Check sheet for the modelled part. Datum: model origin and axes. Units: mm. Give positions to 0.01 mm unless a question says otherwise; leave off trailing zeros. Order: outer loops, then holes, each group sorted by start corner. A loop starts at its lowest first (then second) coordinate and runs counter-clockwise, first axis right, second up. Notation, with made-up numbers: (-17.5, 58) - (11.5, 58) arc R19 cw to (11.5, 79) - close; hole circle Ø1 at (8.25, -25.75). An arc over 180 degrees is marked (long way). Answer in a Markdown table with one row per item.
Autodesk Inventor part; units mm, degrees
ref_plane "YZ Plane" through (0, 0, 0) normal (1, 0, 0) x (0, 1, 0)
ref_plane "XZ Plane" through (0, 0, 0) normal (0, 1, 0) x (-1, 0, 0)
ref_plane "XY Plane" through (0, 0, 0) normal (0, 0, 1) x (1, 0, 0)
sketch "Sketch1" plane through (0, 0, 0) normal (0, 1, 0) x (-1, 0, 0)
  line L0 (-40, 50) -> (40, 50)
  line L1 (40, 50) -> (40, -50)
  line L2 (40, -50) -> (-40, -50)
  line L3 (-40, -50) -> (-40, 50)
  line L4 (-40, 50) -> (40, -50) construction
  line L5 (40, 50) -> (-40, -50) construction
  circle A0 centre (34.29, 45.72) radius 2
  line L6 (-34.29, 45.72) -> (34.29, 45.72) construction
  line L7 (34.29, 45.72) -> (34.29, -45.72) construction
  line L8 (34.29, -45.72) -> (-34.29, -45.72) construction
  line L9 (-34.29, -45.72) -> (-34.29, 45.72) construction
  line L10 (-34.29, 45.72) -> (34.29, -45.72) construction
  line L11 (34.29, 45.72) -> (-34.29, -45.72) construction
  circle A1 centre (34.29, -45.72) radius 2
  circle A2 centre (-34.29, -45.72) radius 2
  circle A3 centre (-34.29, 45.72) radius 2
  point P0 (0, 0)
  dimension "d0" = 100
  dimension "d1" = 80
  dimension "d2" = 4
  dimension "d15" = 91.44
  dimension "d16" = 68.58
  dimension "d17" = 4
  dimension "d18" = 4
  dimension "d19" = 4
extrude "Extrusion1" add sketch "Sketch1" along normal blind 2
properties part number "PCB" material "ABS Plastic"
(1) Cross-section at A-A, the plane x = -34.29. Record the cut outline in (y, z).
Geometry says:
| item | result |
|---|---|
| outline | (0, -50) - (2, -50) - (2, -47.72) - (0, -47.72) - close; (0, -43.72) - (2, -43.72) - (2, 43.72) - (0, 43.72) - close; (0, 47.72) - (2, 47.72) - (2, 50) - (0, 50) - close |
(2) Mould release check, pull along Z, two halves, no side actions. Record for faces 1 (the flat face through (1, 1, 50)), 2 (the flat face through (40, 1, -1)), 3 (the cylindrical face through (-34.03, 0.986, 43.737)): pulls with the +Z half, pulls with the -Z half, needs draft (parallel to the pull), parting line crosses it, or undercut.
Geometry says:
| item | result |
|---|---|
| face 1 | pulls with the +Z half |
| face 2 | needs draft |
| face 3 | undercut |
(3) Thickness scan on L1, parallel to Z at x = -34.29, y = 0.65; L2, parallel to Z at x = 36, y = 1.2. Record the ranges inside material, lowest first.
Geometry says:
| item | result |
|---|---|
| L1 | -50 to -47.72, -43.72 to 43.72, 47.72 to 50 |
| L2 | -50 to -46.76, -44.68 to 44.68, 46.76 to 50 |
(4) Gauge pin test, flat end, axial feed: P1, Ø3.5, axis at x = -34.29, z = -45.72, coming from the -Y side. Record the tip position at first contact, or that the pin passes through.
Geometry says:
| item | result |
|---|---|
| P1 | through |
(5) Cross-section at B-B, the plane z = -45.72. Record the cut outline in (x, y).
Geometry says:
| item | result |
|---|---|
| outline | (-40, 0) - (-36.29, 0) - (-36.29, 2) - (-40, 2) - close; (-32.29, 0) - (32.29, 0) - (32.29, 2) - (-32.29, 2) - close; (36.29, 0) - (40, 0) - (40, 2) - (36.29, 2) - close |
